Autodesk Inventor part; units mm, degrees
ref_plane "工作平面2" through (90, 10, 110) normal (0.1219, 0.9925, 0) x (0, 0, -1)
ref_plane "YZ Plane" through (0, 0, 0) normal (1, 0, 0) x (0, 1, 0)
ref_plane "XZ Plane" through (0, 0, 0) normal (0, 1, 0) x (-1, 0, 0)
sketch "草圖1" plane through (0, 0, 0) normal (0, 1, 0) x (-1, 0, 0)
  line L0 (90, 110) -> (-90, 110)
  line L1 (-90, 110) -> (-90, -110)
  line L2 (-90, -110) -> (90, -110)
  line L3 (90, -110) -> (90, 110)
  line L4 (90, 110) -> (-90, -110) construction
  line L5 (-90, 110) -> (90, -110) construction
  point P0 (0, 0)
  dimension "d0" = 180
  dimension "d1" = 220
extrude "擠出1" add sketch "草圖1" along normal blind 10
sketch "草圖3" plane through (0, 10, 0) normal (0, 1, 0) x (1, 0, 0)
  line L0 (90, -110) -> (90, 110)
  line L1 (90, 110) -> (-90, 110)
  line L2 (-90, 110) -> (-90, -110)
  line L3 (-90, -110) -> (90, -110)
  point P0 (0, 0)
extrude "擠出2" add sketch "草圖3" along normal blind 100
sketch "草圖4" plane through (90, 0, 110) normal (1, 0, 0) x (0, 0, -1)
  line L0 (0, 0) -> (220, 0)
  line L1 (220, 0) -> (220, 110)
  line L2 (0, 110) -> (220, 110)
  line L3 (0, 0) -> (0, 110)
  line L4 (0, 0) -> (0, 110)
  line L5 (0, 10) -> (220, 10)
  point P0 (110, 0)
  dimension "d7" = 10
ref_plane "工作平面2" through (90, 10, 110) normal (0.1219, 0.9925, 0) x (0, 0, -1)
split "分割1" plane through (90, 10, 110) removes the side toward (0.1219, 0.9925, 0)
sketch "草圖5" plane through (0, 0, 0) normal (0, -1, 0) x (1, 0, 0)
  line L0 (-75, -75) -> (75, -75) construction
  line L1 (75, -75) -> (75, 75) construction
  line L2 (75, 75) -> (-75, 75) construction
  line L3 (-75, 75) -> (-75, -75) construction
  line L4 (-75, -75) -> (75, 75) construction
  line L5 (75, -75) -> (-75, 75) construction
  point P0 (0, 0)
  dimension "d9" = 150
  dimension "d10" = 150
hole "孔1" at (-75, 0, -75) at (75, 0, -75) at (75, 0, 75) at (-75, 0, 75) direction (0, 1, 0) diameter 4.2 depth 4
sketch "草圖6" plane through (-75, 4, -75) normal (0, -1, 0) x (1, 0, 0)
  circle A0 centre (0, 150) radius 2.1
  circle A1 centre (150, 150) radius 2.1
  circle A2 centre (150, 0) radius 2.1
  circle A3 centre (0, 0) radius 2.1
  circle A4 centre (0, 0) radius 2.1
  circle A5 centre (150, 0) radius 2.1
  circle A6 centre (0, 150) radius 2.1
  point P0 (75, 75)
hole "孔2" at (-75, 4, -75) at (75, 4, -75) at (75, 4, 75) at (-75, 4, 75) direction (0, 1, 0) diameter 11 end through all
sketch "草圖7" plane through (90, 10, 110) normal (0.1219, 0.9925, 0) x (0.9925, -0.1219, 0)
  line L0 (-163.1105, 15) -> (-13.1105, 15)
  line L1 (-13.1105, 15) -> (-13.1105, 205)
  line L2 (-13.1105, 205) -> (-163.1105, 205)
  line L3 (-163.1105, 205) -> (-163.1105, 15)
  line L4 (-163.1105, 15) -> (-13.1105, 205) construction
  line L5 (-13.1105, 15) -> (-163.1105, 205) construction
  point P0 (-88.1105, 110)
  dimension "d25" = 150
  dimension "d26" = 190
hole "孔3" at (-71.8947, 29.8782, 95) at (76.9873, 11.5978, 95) at (76.9873, 11.5978, -95) at (-71.8947, 29.8782, -95) direction (-0.1219, -0.9925, 0) diameter 5.5 depth 10 counterbore diameter 8.1 counterbore depth 6
sketch "草圖8" plane through (0, 0, 0) normal (0, -1, 0) x (1, 0, 0)
  line L0 (-62.5, 72.5) -> (62.5, 72.5)
  line L1 (62.5, 72.5) -> (62.5, -72.5)
  line L2 (62.5, -72.5) -> (-62.5, -72.5)
  line L3 (-62.5, -72.5) -> (-62.5, 72.5)
  line L4 (-62.5, 72.5) -> (62.5, -72.5) construction
  line L5 (62.5, 72.5) -> (-62.5, -72.5) construction
  point P0 (0, 0)
  dimension "d34" = 125
  dimension "d35" = 145
extrude "擠出3" cut sketch "草圖8" against normal through all
fillet "圓角2" radius 20 8 edges at (-90, 16.0506, 110) (90, 5, 110) (90, 5, -110) (-90, 16.0506, -110) (-62.5, 14.3623, -72.5) (-62.5, 14.3623, 72.5) (62.5, 6.6883, 72.5) (62.5, 6.6883, -72.5)
equation "\"d9\" = d10"
properties part number "頸部桌面轉接件"
CAD build for the part. Positions are in the model's coordinates, mm. A direction names the side the tool comes from. Round coordinates to 2 decimals unless told otherwise and drop trailing zeros. Loops run counter-clockwise (first coordinate to the right, second up) from the corner with the lowest first, then second, coordinate; pieces in that order, holes last.
(1) Drop flat-ended pins along their axis: pin 1 (12.5 mm diameter, centred on x = 75, z = -75, fed in from +Y); pin 2 (12.5 mm diameter, centred on x = -75, z = -75, fed in from +Y); pin 3 (12 mm diameter, centred on x = 66.5, z = 32, fed in from -Y); pin 4 (9 mm diameter, centred on x = 76, z = 73.5, fed in from +Y). Give the stop position or say it passes through.
(2) Wall check: line 1 along X through (y, z) = (1, 75); line 2 along Z through (x, y) = (17.5, 1); line 3 along Z through (x, y) = (-75, 14). Give the ranges that are in metal, low to high.
(3) Cut at B-B (x = 32). Give the cut face in (y, z), plus the area to 3 significant figures.
(4) Which spindle directions (+Z, -Z, +X, -X, +Y, -Y) get a long thin tool onto all of the face, cutting with end or side? Do faces 4 (the flat face through (-62.5, 14, -1)), 5 (the cylindrical face through (83.986, 4.931, 104.297)), 6 (the flat face through (-75.1, 4, 72.6)). Say none if no direction does.
(5) Two-plate mould, pull along Z, no slides. Class faces 1 (the cylindrical face through (-84.297, 15.826, -103.986)), 2 (the flat face through (-90, 16, -1)), 3 (the flat face through (74.9, 4, 72.6)): +Z half, -Z half, draft (parallel to the pull), parting line (faces both ways), or undercut.
(6) Cut at A-A (z = 47). Give the cut face in (x, y).
Findings below:
1. pin 1: stops at y = 12.61
1. pin 2: stops at y = 31.03
1. pin 3: stops at y = 0
1. pin 4: stops at y = 12.01
2. line 1: x = -90 to -77.1, -72.9 to 72.9, 77.1 to 90
2. line 2: z = -110 to -72.5, 72.5 to 110
2. line 3: z = -109.36 to -80.5, -69.5 to 69.5, 80.5 to 109.36
3. outline: (0, -110) - (17.12, -110) - (17.12, -72.5) - (0, -72.5) - close; (0, 72.5) - (17.12, 72.5) - (17.12, 110) - (0, 110) - close
3. area: 1,280 mm2
4. face 4: +Y, -Y
4. face 5: +Z, +X, +Y, -Y
4. face 6: +Y
5. face 1: -Z half
5. face 2: draft
5. face 3: undercut
6. outline: (-90, 0) - (-62.5, 0) - (-62.5, 28.72) - (-90, 32.1) - close; (62.5, 0) - (90, 0) - (90, 10) - (62.5, 13.38) - close
